Check sheet for the modelled part. Datum: model origin and axes. Units: mm. Face numbers are marked on the shaded views. A direction names the side the tool comes from. Give positions to 0.01 mm unless a question says otherwise; leave off trailing zeros. Order: outer loops, then holes, each group sorted by start corner. A loop starts at its lowest first (then second) coordinate and runs counter-clockwise, first axis right, second up.
```python
from build123d import *

# Parameters (mm, degrees)
SKETCH_1_W          = 17.5
SKETCH_1_H          = 13
EXTRUDE_1_DEPTH     = 6
EXTRUDE_2_DEPTH     = 3
EXTRUDE_3_REACH     = 23.03
SKETCH_3_R          = 1.150331691
EXTRUDE_4_DEPTH     = 3
SKETCH_6_R          = 1.2
CUT_EXTRUDE_1_DEPTH = 5


with BuildPart() as part:
    # Sketch 1 → Extrude 1 (new body)
    with BuildSketch(Plane.XY):
        with Locations((-8.75, 6.5)):
            Rectangle(SKETCH_1_W, SKETCH_1_H)
    extrude(amount=EXTRUDE_1_DEPTH)

    # Sketch 2 → Extrude 2 (add)
    with BuildSketch(Plane(origin=(0, 13, 0), x_dir=(1, 0, 0), z_dir=(0, 1, 0))):
        with BuildLine():
            Line((-12.632855568, 3.5), (-13.25, 0))
            Line((-13.25, 0), (-9.75, 0))
            Line((-9.75, 0), (-10.367144432, 3.5))
            ThreePointArc((-10.367144432, 3.5), (-11.5, 4.450578689), (-12.632855568, 3.5))
        make_face()
        with BuildLine():
            Line((-4.867144432, 3.5), (-4.25, 0))
            Line((-4.25, 0), (-7.75, 0))
            Line((-7.75, 0), (-7.132855568, 3.5))
            ThreePointArc((-7.132855568, 3.5), (-6, 4.450578689), (-4.867144432, 3.5))
        make_face()
    extrude_2 = extrude(amount=-EXTRUDE_2_DEPTH)

    # Mirror 1: Extrude 2 across plane
    add(extrude_2.mirror(Plane.ZX.offset(6.5)))

    # Sketch 3 → Extrude 3 (add, up to next)
    with BuildSketch(Plane(origin=(0, 3, 0), x_dir=(1, 0, 0), z_dir=(0, 1, 0)), mode=Mode.PRIVATE) as extrude_3_sk1:
        with Locations(Location((-11.5, 3.300246998, 0), (0, 0, 10))):
            Circle(SKETCH_3_R)
    extrude_3_tool1 = extrude(extrude_3_sk1.sketch, amount=EXTRUDE_3_REACH, mode=Mode.PRIVATE) - part.part
    # Sketch 3 → Extrude 3 (add, up to next)
    with BuildSketch(Plane(origin=(0, 3, 0), x_dir=(1, 0, 0), z_dir=(0, 1, 0)), mode=Mode.PRIVATE) as extrude_3_sk2:
        with Locations(Location((-6, 3.300246998, 0), (0, 0, 170))):
            Circle(SKETCH_3_R)
    extrude_3_tool2 = extrude(extrude_3_sk2.sketch, amount=EXTRUDE_3_REACH, mode=Mode.PRIVATE) - part.part
    add(extrude_3_tool1.solids().sort_by_distance((-11.5, 3, -3.300247))[0])
    add(extrude_3_tool2.solids().sort_by_distance((-6, 3, -3.300247))[0])

    # Sketch 4 → Extrude 4 (add)
    with BuildSketch(Plane.ZY.offset(17.5)):
        Polygon((0, 11.5), (0, 1.5), (-1, 3.5), (-1, 9.5), align=None)
    extrude_4 = extrude(amount=-EXTRUDE_4_DEPTH)

    # Mirror 2: Extrude 4 across plane
    add(extrude_4.mirror(Plane(origin=(-8.75, 0, 0), x_dir=(0, 0, 1), z_dir=(1, 0, 0))))

    # Sketch 6 → Cut-Extrude 1 (cut)
    with BuildSketch(Plane(origin=(0, 13, 0), x_dir=(1, 0, 0), z_dir=(0, 1, 0))):
        with Locations(Location((-14, -2.5, 0), (0, 0, 270))):
            Circle(SKETCH_6_R)
        with Locations(Location((-3.5, -2.5, 0), (0, 0, 270))):
            Circle(SKETCH_6_R)
    cut_extrude_1 = extrude(amount=-CUT_EXTRUDE_1_DEPTH, mode=Mode.SUBTRACT)

    # Mirror 3: Cut-Extrude 1 across plane
    add(cut_extrude_1.mirror(Plane.ZX.offset(6.5)), mode=Mode.SUBTRACT)


solid = part.part
```
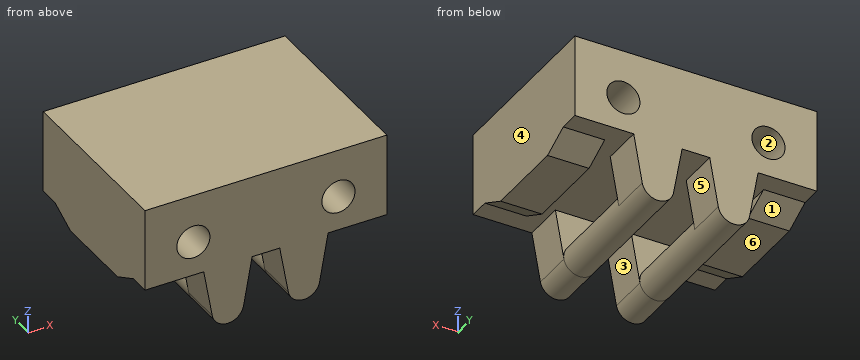
Q1. Material ranges on line 1 (X direction, y = 11.8, z = 2.5); line 2 (X direction, y = 5.5, z = -3.25); line 3 (Y direction, x = -12, z = -2), recorded low to high.
Q2. Sectioned sample at C-C, the plane y = 10.5. Record the cut outline in (x, z).
Q3. Sectioned sample at B-B, the plane x = -6. Record the cut outline in (y, z), plus the area to 3 significant figures.
Q4. Draft check along X on the marked faces 4, 5 and 6. Enter one of: pulls with the +X half, pulls with the -X half, needs draft (parallel to the pull), parting line crosses it, or undercut.
Q5. Sectioned sample at D-D, the plane z = -2.75. Record the cut outline in (x, y).
Q6. Tool access check on the marked faces 1, 2 and 3. Record the directions out of +Z, -Z, +X, -X, +Y, -Y that give a thin tool (end or side, any length) a straight path to the whole face; none if there is none.
Q7. Sectioned sample at A-A, the plane y = 4.75. Record the cut outline in (x, z), plus the area to 3 significant figures.
Q8. Go/stop test with flat-tipped pins: P1, Ø2, axis at x = -14, z = 2.5, coming from the -Y side; P2, Ø1.5, axis at x = -16.5, y = 7, coming from the -Z side; P3, Ø1.9, axis at x = -3.5, z = 2.5, coming from the +Y side. Record where each tip stops, or that it passes through.
Filled in:
1. line 1: x = -17.5 to -15.2, -12.8 to -4.7, -2.3 to 0
1. line 2: x = -12.65 to -10.35, -7.15 to -4.85
1. line 3: y = 0 to 3, 10 to 13
2. outline: (-17.5, -0.5) - (-14.5, -0.5) - (-14.5, 0) - (-13.25, 0) - (-12.63, -3.5) arc R1.15 ccw to (-10.37, -3.5) - (-9.75, 0) - (-7.75, 0) - (-7.13, -3.5) arc R1.15 ccw to (-4.87, -3.5) - (-4.25, 0) - (-3, 0) - (-3, -0.5) - (0, -0.5) - (0, 6) - (-17.5, 6) - close; hole circle Ø2.4 at (-14, 2.5); hole circle Ø2.4 at (-3.5, 2.5)
3. outline: (0, -4.45) - (13, -4.45) - (13, 6) - (0, 6) - close; hole (3, -2.15) - (10, -2.15) - (10, 0) - (3, 0) - close
3. area: 121 mm2
4. face 4: pulls with the +X half
4. face 5: undercut
4. face 6: needs draft
5. outline: (-12.77, 0) - (-10.23, 0) - (-10.23, 3) - (-10.49, 3) - (-10.49, 10) - (-10.23, 10) - (-10.23, 13) - (-12.77, 13) - (-12.77, 10) - (-12.51, 10) - (-12.51, 3) - (-12.77, 3) - close; (-7.27, 0) - (-4.73, 0) - (-4.73, 3) - (-4.99, 3) - (-4.99, 10) - (-4.73, 10) - (-4.73, 13) - (-7.27, 13) - (-7.27, 10) - (-7.01, 10) - (-7.01, 3) - (-7.27, 3) - close
6. face 1: -Z, -X, +Y
6. face 2: +Y
6. face 3: -Z, +Y, -Y
7. outline: (-17.5, -1) - (-14.5, -1) - (-14.5, 0) - (-3, 0) - (-3, -1) - (0, -1) - (0, 6) - (-17.5, 6) - close; circle Ø2.3 at (-11.5, -3.3); circle Ø2.3 at (-6, -3.3); hole circle Ø2.4 at (-14, 2.5); hole circle Ø2.4 at (-3.5, 2.5)
7. area: 110 mm2
8. P1: stops at y = 5
8. P2: stops at z = -1
8. P3: stops at y = 8
